from build123d import *

# Parameters (mm, degrees)
SKETCH_1_R               = 3.6
SKETCH_1_R_2             = 2.8
EXTRUDE_1_DEPTH          = 8.4
SKETCH_2_W               = 8
SKETCH_2_H               = 19.939100818
EXTRUDE_2_DEPTH          = 20
SKETCH_3_W               = 8
SKETCH_3_H               = 20
EXTRUDE_3_DEPTH          = 20
SKETCH_4_W               = 8
SKETCH_4_H               = 14
CUT_EXTRUDE_2_DEPTH      = 18
SKETCH_5_W               = 8
SKETCH_5_H               = 14
CUT_EXTRUDE_3_DEPTH      = 18
SKETCH_6_R               = 1.6
CUT_EXTRUDE_4_DEPTH      = 10
CUT_EXTRUDE_4_DEPTH_BACK = 29


with BuildPart() as part:
    # 草图1 → 凸台-拉伸1 (new body)
    with BuildSketch(Plane.XY):
        Circle(SKETCH_1_R)
        Circle(SKETCH_1_R_2, mode=Mode.SUBTRACT)
    extrude(amount=EXTRUDE_1_DEPTH)

    # 草图2 → 凸台-拉伸2 (add)
    with BuildSketch(Plane(origin=(0, 0, 0), x_dir=(-1, 0, 0), z_dir=(0, 0, -1))):
        Rectangle(SKETCH_2_W, SKETCH_2_H)
    extrude(amount=EXTRUDE_2_DEPTH)

    # 草图3 → 凸台-拉伸3 (add)
    with BuildSketch(Plane.XY.offset(8.4)):
        Rectangle(SKETCH_3_W, SKETCH_3_H)
    extrude(amount=EXTRUDE_3_DEPTH)

    # 草图4 → 切除-拉伸2 (cut)
    with BuildSketch(Plane(origin=(0, 0, -20), x_dir=(-1, 0, 0), z_dir=(0, 0, -1))):
        Rectangle(SKETCH_4_W, SKETCH_4_H)
    extrude(amount=-CUT_EXTRUDE_2_DEPTH, mode=Mode.SUBTRACT)

    # 草图5 → 切除-拉伸3 (cut)
    with BuildSketch(Plane.XY.offset(28.4)):
        Rectangle(SKETCH_5_W, SKETCH_5_H)
    extrude(amount=-CUT_EXTRUDE_3_DEPTH, mode=Mode.SUBTRACT)

    # 草图6 → 切除-拉伸4 (cut, two sides)
    with BuildSketch(Plane(origin=(0, 9.969550409, 0), x_dir=(1, 0, 0), z_dir=(0, 1, 0))) as cut_extrude_4_sk:
        with Locations((0, 17)):
            Circle(SKETCH_6_R)
        with Locations((0, -25.4)):
            Circle(SKETCH_6_R)
    extrude(amount=CUT_EXTRUDE_4_DEPTH, mode=Mode.SUBTRACT)
    extrude(cut_extrude_4_sk.sketch, amount=-CUT_EXTRUDE_4_DEPTH_BACK, mode=Mode.SUBTRACT)


solid = part.part
Geometry: final body of the model. Coordinates: model frame, mm. A direction names the side the tool comes from. Coordinates: 2 decimals unless noted, no trailing zeros. Loops run counter-clockwise (first coordinate to the right, second up) from the corner with the lowest first, then second, coordinate; pieces in that order, holes last. Notation, with made-up numbers: M -37,-8 L -22,-8 A19 ccw -22,13 Z; hole C -12,17 d2. An arc over 180 degrees is marked long. One line per item, written item: value. Start each with the question number.
1) Draft query along Y for faces 1 (the cylindrical face through (-2.8, 0.1, 4.1)), 2 (the flat face through (-4, -7.5, 16.1)), 3 (the flat face through (0, -10, 18)). Return one class per face: released by +Y, released by -Y, zero draft, split by the parting line, or undercut.
2) Cut plane B-B (z = -2.5). Return loops of the section in (x, y).
3) Cut plane A-A (y = -8). Return loops of the section in (x, z).
4) Cut plane C-C (z = -17). Return loops of the section in (x, y).
5) Reachability of faces 4 (the flat face through (0, -7, -11)), 5 (the flat face through (0, 7, 20)), 6 (the flat face through (0, -8, -20)) from +Z, -Z, +X, -X, +Y, -Y: full face, straight path, thin tool, end or side. Return the list, or none.
6) Cut plane D-D (x = 0). Count the separate pieces of the cut face and the enclosed holes in it, then the cut area to 3 significant figures.
7) Material intervals for L1, parallel to Z at x = 0, y = 9; L2, parallel to Z at x = 3.75, y = -7.75; L3, parallel to Z at x = 3.25, y = 3.5, sorted ascending. Write a range as from..to.
8) Pin query (flat end, axial travel): P1, Ø3, axis at x = 0.5, z = -14, coming from the -Y side; P2, Ø1.7, axis at x = -0.5, y = -1, coming from the +Z side; P3, Ø1, axis at y = -2.5, z = 5.5, coming from the +X side. Return the tip coordinate at first contact, or that it passes through.
Evaluation:
1. face 1: undercut
1. face 2: zero draft
1. face 3: released by -Y
2. outline: M -4,-9.97 L 4,-9.97 L 4,-7 L -4,-7 Z; M -4,7 L 4,7 L 4,9.97 L -4,9.97 Z
3. outline: M -4,-20 L 4,-20 L 4,0 L -4,0 Z; M -4,8.4 L 4,8.4 L 4,28.4 L -4,28.4 Z; hole C 0,-17 d3.2; hole C 0,25.4 d3.2
4. outline: M -4,-9.97 L -1.6,-9.97 L -1.6,-7 L -4,-7 Z; M -4,7 L -1.6,7 L -1.6,9.97 L -4,9.97 Z; M 1.6,-9.97 L 4,-9.97 L 4,-7 L 1.6,-7 Z; M 1.6,7 L 4,7 L 4,9.97 L 1.6,9.97 Z
5. face 4: -Z, +X, -X
5. face 5: +Z, +X, -X
5. face 6: -Z, +X, -X, +Y, -Y
6. separate pieces: 5
6. enclosed holes: 1
6. area: 270 mm^2
7. L1: -20..-18.6, -15.4..0, 8.4..23.8, 27..28.4
7. L2: -20..0, 8.4..28.4
7. L3: -2..0, 8.4..10.4
8. P1: y = -9.97
8. P2: z = 10.4
8. P3: x = 2.99
